Geometry check sheet. Reference: the model listing, model coordinates, mm. Face numbers are marked on the shaded views. A direction names the side the tool comes from. Coordinates: 2 decimals unless noted, no trailing zeros. Write each loop counter-clockwise with the first axis right and the second up, starting at its lowest first coordinate (ties: lowest second). Pieces come first, ordered by that corner, then holes. Notation, with made-up numbers: (80.5, 23) - (129.5, 23) arc R29 ccw to (129.5, 54) - close; hole circle Ø7 at (-27.75, 31). An arc over 180 degrees is marked (long way). Answer as a JSON object with one key per item and string values. Group by question number.
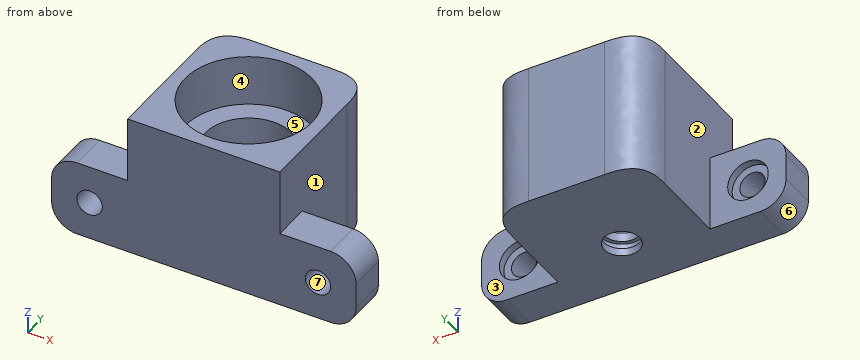
from build123d import *

# Parameters (mm, degrees)
BOSS_EXTRUDE1_DEPTH      = 20
BOSS_EXTRUDE1_DEPTH_BACK = 8
SKETCH1_W                = 30
SKETCH1_H                = 30
FILLET1_SIZE             = 7.5
SKETCH2_R                = 8.5
CUT_EXTRUDE1_DEPTH       = 60
SKETCH3_W                = 15
SKETCH3_H                = 7.5
BOSS_EXTRUDE2_DEPTH      = 15
SKETCH5_W                = 15
SKETCH5_H                = 7.5
BOSS_EXTRUDE4_DEPTH      = 15
SKETCH11_R               = 12.5
CUT_EXTRUDE3_DEPTH       = 10
SKETCH12_R               = 3.5
CUT_EXTRUDE4_DEPTH       = 10
FILLET8_R                = 5
SKETCH15_R               = 4
CUT_EXTRUDE5_DEPTH       = 1.5
SKETCH16_R               = 2.5
CUT_EXTRUDE6_DEPTH       = 12
CUT_EXTRUDE8_START       = -1.5
SKETCH18_R               = 4.25
CUT_EXTRUDE8_DEPTH       = 1.75
CUT_EXTRUDE9_START       = -5
SKETCH18_2_R             = 4.25
CUT_EXTRUDE9_DEPTH       = 1.5


with BuildPart() as part:
    # Sketch1 → Boss-Extrude1 (new, two sides: drawn at the far end of the back side and taken through both)
    with BuildSketch(Plane.XY.offset(-BOSS_EXTRUDE1_DEPTH_BACK)):
        Rectangle(SKETCH1_W, SKETCH1_H)
    extrude(amount=BOSS_EXTRUDE1_DEPTH + BOSS_EXTRUDE1_DEPTH_BACK)

    # Fillet1
    # a fillet whose section is not a circle: 7.5 mm, written as the material it takes off along each edge
    with BuildSketch(Plane(origin=(-15, 15, 38.75), x_dir=(1, 0, 0), z_dir=(0, 0, -1))) as fillet1_piece_1:
        with BuildLine():
            add(Edge.make_bspline([(FILLET1_SIZE, 0), (FILLET1_SIZE * 0.831801948466, 0), (FILLET1_SIZE * 0.663603896932, 0), (FILLET1_SIZE * 0.292893218813, FILLET1_SIZE * 0.0716919198361), (FILLET1_SIZE * 0.0716919198361, FILLET1_SIZE * 0.292893218813), (0, FILLET1_SIZE * 0.663603896932), (0, FILLET1_SIZE * 0.831801948466), (0, FILLET1_SIZE)], knots=[0, 0, 0, 0, 0, 0, 0.5, 0.5, 1, 1, 1, 1, 1, 1], degree=5))
            Line((0, FILLET1_SIZE), (0, 0))
            Line((0, 0), (FILLET1_SIZE, 0))
        make_face()
    extrude(amount=65.5, mode=Mode.SUBTRACT)
    with BuildSketch(Plane(origin=(15, 15, -26.75), x_dir=(0, -1, 0), z_dir=(0, 0, 1))) as fillet1_piece_2:
        with BuildLine():
            add(Edge.make_bspline([(FILLET1_SIZE, 0), (FILLET1_SIZE * 0.831801948466, 0), (FILLET1_SIZE * 0.663603896932, 0), (FILLET1_SIZE * 0.292893218813, -FILLET1_SIZE * 0.0716919198361), (FILLET1_SIZE * 0.0716919198361, -FILLET1_SIZE * 0.292893218813), (0, -FILLET1_SIZE * 0.663603896932), (0, -FILLET1_SIZE * 0.831801948466), (0, -FILLET1_SIZE)], knots=[0, 0, 0, 0, 0, 0, 0.5, 0.5, 1, 1, 1, 1, 1, 1], degree=5))
            Line((0, -FILLET1_SIZE), (0, 0))
            Line((0, 0), (FILLET1_SIZE, 0))
        make_face()
    extrude(amount=65.5, mode=Mode.SUBTRACT)

    # Sketch2 → Cut-Extrude1 (cut)
    with BuildSketch(Plane.XY):
        with Locations(Location((0, 0, 0), (0, 0, 180))):
            Circle(SKETCH2_R)
    extrude(amount=CUT_EXTRUDE1_DEPTH, mode=Mode.SUBTRACT)

    # Sketch3 → Boss-Extrude2 (add)
    with BuildSketch(Plane(origin=(15, 0, 0), x_dir=(0, 0, -1), z_dir=(1, 0, 0))):
        with Locations((0.5, -11.25)):
            Rectangle(SKETCH3_W, SKETCH3_H)
    extrude(amount=BOSS_EXTRUDE2_DEPTH)

    # Sketch5 → Boss-Extrude4 (add)
    with BuildSketch(Plane.ZY.offset(15)):
        with Locations((-0.5, -11.25)):
            Rectangle(SKETCH5_W, SKETCH5_H)
    extrude(amount=BOSS_EXTRUDE4_DEPTH)

    # Sketch11 → Cut-Extrude3 (cut)
    with BuildSketch(Plane.XY.offset(20)):
        Circle(SKETCH11_R)
    extrude(amount=-CUT_EXTRUDE3_DEPTH, mode=Mode.SUBTRACT)

    # Sketch12 → Cut-Extrude4 (cut)
    with BuildSketch(Plane.XY):
        with Locations((0, -3.5)):
            Circle(SKETCH12_R)
    extrude(amount=-CUT_EXTRUDE4_DEPTH, mode=Mode.SUBTRACT)

    # Fillet8
    fillet8_edges = [part.edges().sort_by_distance(p)[0] for p in [
        (30, -11.25, -8),
        (30, -11.25, 7),
        (-30, -11.25, -8),
        (-30, -11.25, 7),
    ]]
    fillet(fillet8_edges, radius=FILLET8_R)

    # Sketch15 → Cut-Extrude5 (cut)
    with BuildSketch(Plane(origin=(0, -7.5, 0), x_dir=(1, 0, 0), z_dir=(0, 1, 0))):
        with Locations(Location((22.5, 0.5, 0), (0, 0, 270))):
            Circle(SKETCH15_R)
        with Locations(Location((-22.5, 0.5, 0), (0, 0, 270))):
            Circle(SKETCH15_R)
    extrude(amount=-CUT_EXTRUDE5_DEPTH, mode=Mode.SUBTRACT)

    # Sketch16 → Cut-Extrude6 (cut)
    with BuildSketch(Plane(origin=(0, -9, 0), x_dir=(1, 0, 0), z_dir=(0, 1, 0))):
        with Locations(Location((-22.5, 0.5, 0), (0, 0, 270))):
            Circle(SKETCH16_R)
        with Locations(Location((22.5, 0.5, 0), (0, 0, 270))):
            Circle(SKETCH16_R)
    extrude(amount=-CUT_EXTRUDE6_DEPTH, mode=Mode.SUBTRACT)

    # Sketch18 → Cut-Extrude8 (cut)
    with BuildSketch(Plane.XY.offset(CUT_EXTRUDE8_START)):
        with Locations((0, -3.5)):
            Circle(SKETCH18_R)
    extrude(amount=-CUT_EXTRUDE8_DEPTH, mode=Mode.SUBTRACT)

    # Sketch18<2> → Cut-Extrude9 (cut)
    with BuildSketch(Plane.XY.offset(CUT_EXTRUDE9_START)):
        with Locations((0, -3.5)):
            Circle(SKETCH18_2_R)
    extrude(amount=-CUT_EXTRUDE9_DEPTH, mode=Mode.SUBTRACT)


solid = part.part
(1) Gauge pin test, flat ends, axial feed: pin 1 (10 mm diameter, centred on x = -21, y = 8, fed in from -Z); pin 2 (5 mm diameter, centred on x = 23, y = -7, fed in from +Z); pin 3 (9.5 mm diameter, centred on x = 1.5, y = -2, fed in from +Z); pin 4 (12.5 mm diameter, centred on x = -2.5, y = 2.5, fed in from +Z). Record the tip position at first contact, or that the pin passes through.
(2) Section check D-D (y = 5.5). Record the cut outline in (x, z).
(3) Set-up check for the marked faces 1, 2 and 3: record each of +Z, -Z, +X, -X, +Y, -Y from which the full face is reachable in a straight line by a thin tool's end or side.
(4) Section check B-B (z = -2.25). Count the separate pieces of the cut face and the enclosed holes in it, and give its area (3 significant figures).
(5) Draft check along Z on the marked faces 4, 5, 6 and 7. Enter one of: +Z half, -Z half, draft (parallel to the pull), parting line (faces both ways), or undercut.
(6) Section check A-A (x = 22.5). Record the cut outline in (y, z), and give its area (3 significant figures).
(7) Material ranges on L1, parallel to Y at x = 0, z = 12.5; L2, parallel to X at y = -8.65, z = -0.5; L3, parallel to Y at x = 0, z = -0.45, recorded low to high. Write a range as [from, to].
Conclusion:
{
 "1": {"pin 1": "passes through", "pin 2": "stops at z = 7", "pin 3": "stops at z = 0", "pin 4": "stops at z = 10"},
 "2": {"outline": "(-15, -8) - (15, -8) - (15, 20) - (11.22, 20) - (11.22, 10) - (6.48, 10) - (6.48, 0) - (-6.48, 0) - (-6.48, 10) - (-11.22, 10) - (-11.22, 20) - (-15, 20) - close"},
 "3": {"face 1": "+Z, +X, +Y", "face 2": "+Z, -X, +Y", "face 3": "+Z, -Z, +X, +Y"},
 "4": {"separate pieces": "3", "enclosed holes": "1", "area": "989 mm^2"},
 "5": {"face 4": "draft", "face 5": "+Z half", "face 6": "-Z half", "face 7": "undercut"},
 "6": {"outline": "(-15, -8) - (-7.5, -8) - (-7.5, -4.5) - (-9, -4.5) - (-9, -3) - (-15, -3) - close; (-15, 2) - (-9, 2) - (-9, 3.5) - (-7.5, 3.5) - (-7.5, 7) - (-15, 7) - close", "area": "70.5 mm^2"},
 "7": {"L1": "y = [-15, -12.5], [12.5, 15]", "L2": "x = [-30, -26.5], [-18.5, 18.5], [26.5, 30]", "L3": "y = [-15, -7], [0, 15]"}
}
